from build123d import *

# Parameters (mm, degrees)
BOSS_EXTRU_4_DEPTH      = 15
ESQUISSE4_R             = 10
ESQUISSE4_W             = 20
ESQUISSE4_H             = 5
ENL_V_MAT_EXTRU_3_DEPTH = 15
ESQUISSE5_R             = 5.5
ENL_V_MAT_EXTRU_4_DEPTH = 50
CONG_10_R               = 20
CONG_11_R               = 20
CONG_12_R               = 20
ESQUISSE6_R             = 5.5
ENL_V_MAT_EXTRU_5_DEPTH = 50
ESQUISSE7_R             = 5.5
ENL_V_MAT_EXTRU_6_DEPTH = 50


with BuildPart() as part:
    # Esquisse1 → Boss.-Extru.4 (new body)
    with BuildSketch(Plane.XY):
        Polygon((60, 0), (60, -15), (8.660254038, -15), (-17.009618943, -59.461524227), (-30, -51.961524227), (-42.990381057, -44.461524227), (-17.320508076, 0), (-42.990381057, 44.461524227), (-30, 51.961524227), (-17.009618943, 59.461524227), (8.660254038, 15), (60, 15), align=None)
    extrude(amount=BOSS_EXTRU_4_DEPTH)

    # Esquisse4 → Enlèv. mat.-Extru.3 (cut)
    with BuildSketch(Plane.XY.offset(15)):
        Circle(ESQUISSE4_R)
        Polygon((-11.339745962, -39.641016151), (-1.339745962, -22.320508076), (-5.669872981, -19.820508076), (-15.669872981, -37.141016151), align=None)
        with Locations((30, 7.5)):
            Rectangle(ESQUISSE4_W, ESQUISSE4_H)
        with Locations((30, -7.5)):
            Rectangle(ESQUISSE4_W, ESQUISSE4_H)
        Polygon((-24.330127019, -32.141016151), (-28.660254038, -29.641016151), (-18.660254038, -12.320508076), (-14.330127019, -14.820508076), align=None)
        Polygon((-28.660254038, 29.641016151), (-18.660254038, 12.320508076), (-14.330127019, 14.820508076), (-24.330127019, 32.141016151), align=None)
        Polygon((-15.669872981, 37.141016151), (-11.339745962, 39.641016151), (-1.339745962, 22.320508076), (-5.669872981, 19.820508076), align=None)
    extrude(amount=-ENL_V_MAT_EXTRU_3_DEPTH, mode=Mode.SUBTRACT)

    # Esquisse5 → Enlèv. mat.-Extru.4 (cut)
    with BuildSketch(Plane(origin=(12.990381057, -7.5, 0), x_dir=(0, 0, -1), z_dir=(0.8660254037844365, -0.500000000000004, 0))):
        with Locations(Location((-7.5, -50, 0), (0, 0, 90))):
            Circle(ESQUISSE5_R)
    extrude(amount=-ENL_V_MAT_EXTRU_4_DEPTH, mode=Mode.SUBTRACT)

    # Congé10
    cong_10_edges = [part.edges().sort_by_distance(p)[0] for p in [
        (8.660254038, -15, 7.5),
    ]]
    fillet(cong_10_edges, radius=CONG_10_R)

    # Congé11
    cong_11_edges = [part.edges().sort_by_distance(p)[0] for p in [
        (8.660254038, 15, 7.5),
    ]]
    fillet(cong_11_edges, radius=CONG_11_R)

    # Congé12
    cong_12_edges = [part.edges().sort_by_distance(p)[0] for p in [
        (-17.320508076, 0, 7.5),
    ]]
    fillet(cong_12_edges, radius=CONG_12_R)

    # Esquisse6 → Enlèv. mat.-Extru.5 (cut)
    with BuildSketch(Plane(origin=(12.990381057, 7.5, 0), x_dir=(0, 0, -1), z_dir=(0.8660254037844445, 0.49999999999998984, 0))):
        with Locations(Location((-7.5, 50, 0), (0, 0, 90))):
            Circle(ESQUISSE6_R)
    extrude(amount=-ENL_V_MAT_EXTRU_5_DEPTH, mode=Mode.SUBTRACT)

    # Esquisse7 → Enlèv. mat.-Extru.6 (cut)
    with BuildSketch(Plane(origin=(0, 15, 0), x_dir=(1, 0, 0), z_dir=(0, 1, 0))):
        with Locations(Location((50, -7.5, 0), (0, 0, 270))):
            Circle(ESQUISSE7_R)
    extrude(amount=-ENL_V_MAT_EXTRU_6_DEPTH, mode=Mode.SUBTRACT)


solid = part.part
Can you work these out from the model? Positions are in its coordinate system, mm. A direction names the side the tool comes from. Round coordinates to 2 decimals unless told otherwise and drop trailing zeros. Write each loop counter-clockwise with the first axis right and the second up, starting at its lowest first coordinate (ties: lowest second). Pieces come first, ordered by that corner, then holes. Notation, with made-up numbers: (26.25, -39) - (80.25, -39) arc R24 ccw to (80.25, -4) - close; hole circle Ø6 at (0.25, -14.75). An arc over 180 degrees is marked (long way). Write each question's results on one line, items separated by ' | '. Start each with the question number.
1) Suppose I cut it at A-A (x = 22.5). List the corners of the cut face in (y, z) for me.
2) Suppose I cut it at C-C (x = 50). List the corners of the cut face in (y, z) for me.
3) Suppose I cut it at D-D (y = -28). List the corners of the cut face in (x, z) for me.
4) Please list where these lines run through material, in increasing order: line 1 (Y direction, x = 26, z = 11); line 2 (X direction, y = 0.5, z = 7.5); line 3 (X direction, y = 7.75, z = 7.5).
5) For pin 1 Ø4 at (y, z) = (8, 5) entering from -X; pin 2 Ø4.5 at (x, z) = (35, 9) entering from +Y; pin 3 Ø1.5 at (x, z) = (-1, 4) entering from +Y; pin 4 Ø1.5 at (x, y) = (-28, -16) entering from +Z, each with a flat end and sliding along its axis, tell me the tip position at first contact or that it passes through.
6) Suppose I cut it at B-B (y = 0). List the corners of the cut face in (x, z) for me.
7) We'd pull the mould along X, two halves only. Please class faces 3 (the flat face through (40, 15, 7)), 4 (the flat face through (20, 7, 8)), 5 (the cylindrical face through (10.33, 17.61, 7.6)), 6 (the flat face through (-32.903, 26.99, 7.395)): released by +X, released by -X, zero draft, split by the parting line, or undercut.
8) Which directions (+Z, -Z, +X, -X, +Y, -Y) give clear straight access to the entire face, cutting with the end or side of a thin tool? Please do faces 1 (the flat face through (-26.46, 30.91, 7.6)), 2 (the cylindrical face through (10.33, -17.61, 7.6)).
Here are the results:
1) outline: (-15, 0) - (-10, 0) - (-10, 15) - (-15, 15) - close; (-5, 0) - (5, 0) - (5, 15) - (-5, 15) - close; (10, 0) - (15, 0) - (15, 15) - (10, 15) - close
2) outline: (-15, 0) - (15, 0) - (15, 2) - (-15, 2) - close; (-15, 13) - (15, 13) - (15, 15) - (-15, 15) - close
3) outline: (-33.49, 0) - (-27.71, 0) - (-27.71, 15) - (-33.49, 15) - close; (-21.94, 0) - (-10.39, 0) - (-10.39, 15) - (-21.94, 15) - close; (-4.62, 0) - (1.15, 0) - (1.15, 15) - (-4.62, 15) - close
4) line 1: y = -15 to -10, -5 to 5, 10 to 15 | line 2: x = -20.42 to -9.99, 9.99 to 44.5, 55.5 to 60 | line 3: x = -21.98 to -6.32, 6.32 to 20, 40 to 44.5, 55.5 to 60
5) pin 1: stops at x = -23.09 | pin 2: stops at y = 15 | pin 3: stops at y = 33.03 | pin 4: passes through
6) outline: (-20.41, 0) - (-10, 0) - (-10, 15) - (-20.41, 15) - close; (10, 0) - (60, 0) - (60, 15) - (10, 15) - close; hole circle Ø11 at (50, 7.5)
7) face 3: zero draft | face 4: undercut | face 5: released by +X | face 6: released by -X
8) face 1: +Z, -Z | face 2: +Z, -Z, +X, -Y
